from build123d import *

# Parameters (mm, degrees)
SKETCH1_W           = 560.57
SKETCH1_H           = 889
BOSS_EXTRUDE1_DEPTH = 44.45
CUT_EXTRUDE2_DEPTH  = 381


with BuildPart() as part:
    # Sketch1 → Boss-Extrude1 (new body)
    with BuildSketch(Plane.XY):
        with Locations((280.285, -444.5)):
            Rectangle(SKETCH1_W, SKETCH1_H)
    extrude(amount=BOSS_EXTRUDE1_DEPTH)

    # Sketch2 → Cut-Extrude2 (cut, symmetric)
    with BuildSketch(Plane(origin=(0, -444.5, 0), x_dir=(1, 0, 0), z_dir=(0, 1, 0))):
        with BuildLine():
            Line((75.435663802, -10), (75.435663802, 0))
            Line((75.435663802, 0), (111.564336198, 0))
            Line((111.564336198, 0), (111.564336198, -10))
            ThreePointArc((111.564336198, -10), (93.5, -23.001673148), (75.435663802, -10))
        make_face()
        with BuildLine():
            Line((168.935663802, -10), (168.935663802, 0))
            Line((168.935663802, 0), (205.064336198, 0))
            Line((205.064336198, 0), (205.064336198, -10))
            ThreePointArc((205.064336198, -10), (187, -23.001673148), (168.935663802, -10))
        make_face()
    cut_extrude2 = extrude(amount=CUT_EXTRUDE2_DEPTH, both=True, mode=Mode.SUBTRACT)

    # Mirror1: Cut-Extrude2 across plane
    add(cut_extrude2.mirror(Plane.ZY.offset(-280.285)), mode=Mode.SUBTRACT)


solid = part.part
Input: part model. Units: mm. Frame: model coordinates. A direction names the side the tool comes from. Give positions to 0.01 mm unless a question says otherwise; leave off trailing zeros. Loops run counter-clockwise (first coordinate to the right, second up) from the corner with the lowest first, then second, coordinate; pieces in that order, holes last. Notation, with made-up numbers: (-6.5, -24) -> (1.5, -24) arc R23 ccw to (1.5, -8) -> close; hole circle Ø8 at (0.25, -34). An arc over 180 degrees is marked (long way). Answer as a JSON object with one key per item and string values. Group by question number.
Item 1: Pin query (flat end, axial travel): P1, Ø7, axis at x = 458.5, z = 10.5, coming from the +Y side; P2, Ø3, axis at x = 378, y = -693, coming from the -Z side. Return the tip coordinate at first contact, or that it passes through.
Item 2: Reachability of faces 4 (the flat face through (276, -438, 0)), 5 (the flat face through (94, -63.5, 9)) from +Z, -Z, +X, -X, +Y, -Y: full face, straight path, thin tool, end or side. Return the list, or none.
Item 3: Cut plane A-A, the plane y = -613.5. Return the cut outline in (x, z), and give its area (3 significant figures).
Item 4: Line query: probe 1 along X at (y, z) = (-336, 3.5); probe 2 along X at (y, z) = (-664, 10.5); probe 3 along Y at (x, z) = (473, 16). Output: solid intervals per line, ascending.
Item 5: Pull-direction query (Y, two-part tool) for faces 1 (the flat face through (560.57, -451, 22)), 2 (the flat face through (276, 0, 22)), 3 (the flat face through (467, -825.5, 9)); classes: released by +Y, released by -Y, zero draft, split by the parting line, or undercut.
Checks:
{
 "1": {"P1": "stops at y = 0", "P2": "stops at z = 22.06"},
 "2": {"face 4": "-Z, +X, -X, +Y, -Y", "face 5": "-Z"},
 "3": {"outline": "(0, 0) -> (75.44, 0) -> (75.44, 10) arc R19.05 cw to (111.56, 10) -> (111.56, 0) -> (168.94, 0) -> (168.94, 10) arc R19.05 cw to (205.06, 10) -> (205.06, 0) -> (355.51, 0) -> (355.51, 10) arc R19.05 cw to (391.63, 10) -> (391.63, 0) -> (449.01, 0) -> (449.01, 10) arc R19.05 cw to (485.13, 10) -> (485.13, 0) -> (560.57, 0) -> (560.57, 44.45) -> (0, 44.45) -> close", "area": "22,100 mm²"},
 "4": {"probe 1": "x = 0 to 75.44, 111.56 to 168.94, 205.06 to 355.51, 391.63 to 449.01, 485.13 to 560.57", "probe 2": "x = 0 to 75.61, 111.39 to 169.11, 204.89 to 355.68, 391.46 to 449.18, 484.96 to 560.57", "probe 3": "y = -889 to -825.5, -63.5 to 0"},
 "5": {"face 1": "zero draft", "face 2": "released by +Y", "face 3": "undercut"}
}
